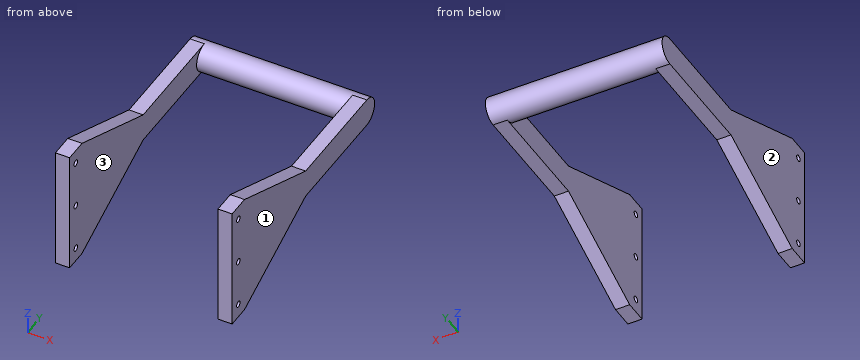
from build123d import *

# Parameters (mm, degrees)
SKETCH_2_W          = 10
SKETCH_2_H          = 88
EXTRUDE_1_DEPTH     = 16
EXTRUDE_1_2_DEPTH   = 16
SKETCH_3_W          = 10
SKETCH_3_H          = 20
EXTRUDE_2_DEPTH     = 158
SKETCH_4_R          = 10
EXTRUDE_3_DEPTH     = 124.5
SKETCH_5_R          = 2.2
CUT_EXTRUDE_1_DEPTH = 126
EXTRUDE_4_DEPTH     = 10
EXTRUDE_5_DEPTH     = 10


with BuildPart() as part:
    # Sketch 2 → Extrude 1 (new body)
    with BuildSketch(Plane(origin=(0, 0, 0), x_dir=(1, 0, 0), z_dir=(0, 1, 0))):
        with Locations((-57.25, 0)):
            Rectangle(SKETCH_2_W, SKETCH_2_H)
    extrude(amount=EXTRUDE_1_DEPTH)



with BuildPart() as body_2:
    # Sketch 2 → Extrude 1 2 (new body)
    with BuildSketch(Plane(origin=(0, 0, 0), x_dir=(1, 0, 0), z_dir=(0, 1, 0))):
        with Locations((57.25, 0)):
            Rectangle(SKETCH_2_W, SKETCH_2_H)
    extrude(amount=EXTRUDE_1_2_DEPTH)


with BuildPart() as part_1:
    add(part.part)

    add(body_2.part)  # Extrude 2 merges body 2
    # Sketch 3 → Extrude 2 (add)
    with BuildSketch(Plane(origin=(0, 16, 0), x_dir=(1, 0, 0), z_dir=(0, 1, 0))):
        with Locations((-57.25, 0)):
            Rectangle(SKETCH_3_W, SKETCH_3_H)
        with Locations((57.25, 0)):
            Rectangle(SKETCH_3_W, SKETCH_3_H)
    extrude(amount=EXTRUDE_2_DEPTH)

    # Sketch 4 → Extrude 3 (add)
    with BuildSketch(Plane.ZY.offset(62.25)):
        with Locations((0, 174)):
            Circle(SKETCH_4_R)
    extrude(amount=-EXTRUDE_3_DEPTH)

    # Sketch 5 → Cut-Extrude 1 (cut)
    with BuildSketch(Plane.ZY.offset(62.25)):
        with Locations((0, 8)):
            Circle(SKETCH_5_R)
        with Locations((-34, 8)):
            Circle(SKETCH_5_R)
        with Locations((34, 8)):
            Circle(SKETCH_5_R)
    extrude(amount=-CUT_EXTRUDE_1_DEPTH, mode=Mode.SUBTRACT)

    # Sketch 6 → Extrude 4 (add)
    with BuildSketch(Plane.ZY.offset(62.25)):
        Polygon((-44, 16), (-10, 95), (-10, 16), align=None)
        Polygon((44, 16), (10, 95), (10, 16), align=None)
    extrude(amount=-EXTRUDE_4_DEPTH)

    # Sketch 7 → Extrude 5 (add)
    with BuildSketch(Plane(origin=(62.25, 0, 0), x_dir=(0, 0, -1), z_dir=(1, 0, 0))):
        Polygon((-44, 16), (-10, 95), (-10, 16), align=None)
        Polygon((44, 16), (10, 95), (10, 16), align=None)
    extrude(amount=-EXTRUDE_5_DEPTH)


solid = part_1.part
Verification items for the finished model (mm, model axes). Face numbers are marked on the shaded views. Give positions to 0.01 mm unless a question says otherwise; leave off trailing zeros. Write each loop counter-clockwise with the first axis right and the second up, starting at its lowest first coordinate (ties: lowest second). Pieces come first, ordered by that corner, then holes. Notation, with made-up numbers: (54.25, 5.5) -> (64.25, 5.5) arc R16 ccw to (64.25, 17.5) -> close; hole circle Ø8 at (-27.75, 3.25). An arc over 180 degrees is marked (long way). Use CSV: the item, a comma, the result in double quotes.
(1) Sectioned sample at B-B (y = 8). Give the number of separate pieces and of enclosed holes in the cut face, plus the area to 3 significant figures.
Derived:
separate pieces,"8"
enclosed holes,"0"
area,"1,500 mm^2"
(2) Go/stop test with flat-tipped pins: pin 1 (10 mm diameter, centred on y = 95, z = 20.5, fed in from +X); pin 2 (11 mm diameter, centred on x = 56, y = 117.5, fed in from -Z); pin 3 (5 mm diameter, centred on y = 8, z = -34, fed in from -X); pin 4 (5 mm diameter, centred on x = 38, z = 2.5, fed in from -Y). Record where each tip stops, or that it passes through.
Derived:
pin 1,"passes through"
pin 2,"stops at z = -10"
pin 3,"stops at x = -62.25"
pin 4,"stops at y = 164"
(3) Sectioned sample at D-D (z = -18). Record the cut outline in (x, y), plus the area to 3 significant figures.
Derived:
outline,"(-62.25, 0) -> (-52.25, 0) -> (-52.25, 76.41) -> (-62.25, 76.41) -> close; (52.25, 0) -> (62.25, 0) -> (62.25, 76.41) -> (52.25, 76.41) -> close"
area,"1,530 mm^2"
(4) Material ranges on L1, parallel to X at y = 58, z = 8.5; L2, parallel to Y at x = -57, z = 0; L3, parallel to Z at x = -56.5, y = 10, recorded low to high.
Derived:
L1,"x = -62.25 to -52.25, 52.25 to 62.25"
L2,"y = 0 to 5.8, 10.2 to 184"
L3,"z = -44 to -34.92, -33.08 to -0.92, 0.92 to 33.08, 34.92 to 44"
(5) Sectioned sample at C-C (y = 141). Record the cut outline in (x, z).
Derived:
outline,"(-62.25, -10) -> (-52.25, -10) -> (-52.25, 10) -> (-62.25, 10) -> close; (52.25, -10) -> (62.25, -10) -> (62.25, 10) -> (52.25, 10) -> close"
(6) Release check for a two-part mould opening along X. For the marked faces 1, 2 and 3 record: +X half, -X half, draft (parallel to the pull), parting line (faces both ways), or undercut.
Derived:
face 1,"+X half"
face 2,"-X half"
face 3,"undercut"
(7) Sectioned sample at A-A (z = 0). Record the cut outline in (x, y).
Derived:
outline,"(-62.25, 0) -> (-52.25, 0) -> (-52.25, 5.8) -> (-62.25, 5.8) -> close; (-62.25, 10.2) -> (-52.25, 10.2) -> (-52.25, 164) -> (52.25, 164) -> (52.25, 10.2) -> (62.25, 10.2) -> (62.25, 184) -> (-62.25, 184) -> close; (52.25, 0) -> (62.25, 0) -> (62.25, 5.8) -> (52.25, 5.8) -> close"
